from build123d import *

# Parameters (mm, degrees)
F1_DEPTH = 7.5
F3_DEPTH = 15
F4_R     = 2
F5_DEPTH = 27.837
F6_R     = 5


with BuildPart() as f1:
    # F0 (on Right) → F1 (new body, symmetric)
    with BuildSketch(Plane.YZ):
        with BuildLine():
            ThreePointArc((12.3245305001, 6.4665811641), (10.2993352496, 7.0979164137), (9.668, 5.0727211632))
            ThreePointArc((9.668, 5.0727211632), (0, -10.918), (-9.668, 5.0727211632))
            ThreePointArc((-9.668, 5.0727211632), (-10.2993352496, 7.0979164137), (-12.3245305001, 6.4665811641))
            ThreePointArc((-12.3245305001, 6.4665811641), (0, -13.918), (12.3245305001, 6.4665811641))
        make_face()
    extrude(amount=F1_DEPTH, both=True)

    # F2 (on face) → F3 (join, through all)
    with BuildSketch(Plane.YZ.offset(7.5)):
        with BuildLine():
            ThreePointArc((13.918, 0), (0, -13.918), (-13.918, 0))
            Line((-13.918, 0), (-13.918, -52.25))
            Line((-13.918, -52.25), (-7.75, -52.25))
            Line((-7.75, -52.25), (-7.75, -39.5))
            Line((-7.75, -39.5), (7.75, -39.5))
            Line((7.75, -39.5), (7.75, -52.25))
            Line((7.75, -52.25), (13.918, -52.25))
            Line((13.918, -52.25), (13.918, 0))
        make_face()
        with BuildLine():
            Line((-10.918, -36.5), (-10.918, -10.1658251018))
            ThreePointArc((-10.918, -10.1658251018), (0, -14.918), (10.918, -10.1658251018))
            Line((10.918, -10.1658251018), (10.918, -36.5))
            Line((10.918, -36.5), (-10.918, -36.5))
        make_face(mode=Mode.SUBTRACT)
    extrude(amount=-F3_DEPTH)

    # F4 (on face) → F5 (cut, through all)
    with BuildSketch(Plane(origin=(0, 13.918, 0), x_dir=(-1, 0, 0), z_dir=(0, 1, 0))):
        with Locations((0, -44.75)):
            Circle(F4_R)
    extrude(amount=-F5_DEPTH, mode=Mode.SUBTRACT)

    # F6
    f6_edges = [f1.edges().sort_by_distance(p)[0] for p in [
        (7.5, -10.834, -52.25),
        (-7.5, -10.834, -52.25),
        (7.5, 10.834, -52.25),
        (-7.5, 10.834, -52.25),
        (0, -10.918, -10.165825),
        (0, 10.918, -10.165825),
        (0, -10.918, -36.5),
        (0, 10.918, -36.5),
    ]]
    fillet(f6_edges, radius=F6_R)


solid = f1.part
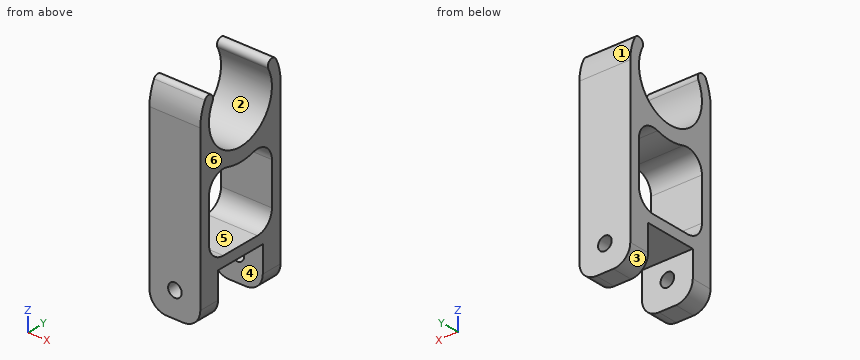
Here's how the part is built. I have some questions about the finished solid (model axes, mm). Face numbers are marked on the shaded views. A direction names the side the tool comes from. Coordinates: 2 decimals unless noted, no trailing zeros. Write each loop counter-clockwise with the first axis right and the second up, starting at its lowest first coordinate (ties: lowest second). Pieces come first, ordered by that corner, then holes.
Item 1: On a 3-axis mill with a long thin cutter (end or side, diameter ignored), from which of +Z, -Z, +X, -X, +Y, -Y can I reach the whole of each face in a straight line? I mean the marked faces 4, 5 and 6. Say none if no direction works.
Item 2: I want a section at A-A on z = -40.5. Write out the boundary of the cut face in (x, y), and give its area (3 significant figures).
Item 3: If I drill on line 1 (Y direction, x = -4, z = -35); line 2 (Y direction, x = -5.5, z = -47.5); line 3 (Z direction, x = 3.25, y = 0), over which ranges is the centre line in solid material (lowest first)?
Item 4: Will these pins go through, and if not, where does the flat tip stop? pin 1 (3 mm diameter, centred on x = -4, y = 2.5, fed in from +Z); pin 2 (4 mm diameter, centred on x = 1, y = 5.5, fed in from +Z); pin 3 (1 mm diameter, centred on x = 1.5, y = 1.5, fed in from -Z).
Item 5: I want a section at C-C on y = 0. Write out the boundary of the cut face in (x, z).
Item 6: I want a section at D-D on x = -4. Write out the boundary of the cut face in (y, z), and give its area (3 significant figures).
Item 7: I want a section at B-B on x = 0. Write out the boundary of the cut face in (y, z), and give its area (3 significant figures).
Item 8: If we mould it in two halves opening along Y, with no side actions, what happens to the marked faces 1, 2 and 3? For each: +Y half, -Y half, draft (parallel to the pull), parting line (faces both ways), or undercut.
Findings below:
1. face 4: -Z, +X, -X
1. face 5: +X, -X
1. face 6: +Z, -Z, +X, +Y, -Y
2. outline: (-7.5, -13.92) - (7.5, -13.92) - (7.5, -7.75) - (-7.5, -7.75) - close; (-7.5, 7.75) - (7.5, 7.75) - (7.5, 13.92) - (-7.5, 13.92) - close
2. area: 185 mm2
3. line 1: y = -13.92 to -9.49, 9.49 to 13.92
3. line 2: y = -13.92 to -7.75, 7.75 to 13.92
3. line 3: z = -39.5 to -36.5, -14.92 to -10.92
4. pin 1: stops at z = -10.16
4. pin 2: stops at z = -7.93
4. pin 3: stops at z = -39.5
5. outline: (-7.5, -39.5) - (7.5, -39.5) - (7.5, -36.5) - (-7.5, -36.5) - close; (-7.5, -14.92) - (7.5, -14.92) - (7.5, -10.92) - (-7.5, -10.92) - close
6. outline: (-13.92, -52.02) - (-7.75, -52.02) - (-7.75, -39.5) - (7.75, -39.5) - (7.75, -52.02) - (13.92, -52.02) - (13.92, 0) arc R13.92 ccw to (12.32, 6.47) arc R1.5 ccw to (9.67, 5.07) arc R10.92 cw (long way) to (-9.67, 5.07) arc R1.5 ccw to (-12.32, 6.47) arc R13.92 ccw to (-13.92, 0) - close; hole (-10.92, -31.5) arc R5 ccw to (-5.92, -36.5) - (5.92, -36.5) arc R5 ccw to (10.92, -31.5) - (10.92, -19.02) arc R5 ccw to (4.43, -14.24) arc R14.92 cw to (-4.43, -14.24) arc R5 ccw to (-10.92, -19.02) - close
6. area: 647 mm2
7. outline: (-13.92, -52.25) - (-7.75, -52.25) - (-7.75, -46.75) - (-13.92, -46.75) - close; (-13.92, -42.75) - (-7.75, -42.75) - (-7.75, -39.5) - (7.75, -39.5) - (7.75, -42.75) - (13.92, -42.75) - (13.92, 0) arc R13.92 ccw to (12.32, 6.47) arc R1.5 ccw to (9.67, 5.07) arc R10.92 cw (long way) to (-9.67, 5.07) arc R1.5 ccw to (-12.32, 6.47) arc R13.92 ccw to (-13.92, 0) - close; (7.75, -52.25) - (13.92, -52.25) - (13.92, -46.75) - (7.75, -46.75) - close; hole (-10.92, -31.5) arc R5 ccw to (-5.92, -36.5) - (5.92, -36.5) arc R5 ccw to (10.92, -31.5) - (10.92, -19.02) arc R5 ccw to (4.43, -14.24) arc R14.92 cw to (-4.43, -14.24) arc R5 ccw to (-10.92, -19.02) - close
7. area: 600 mm2
8. face 1: +Y half
8. face 2: undercut
8. face 3: draft
